For this review, take the finished solid that the model builds, in its own axes (mm). A direction names the side the tool comes from. Round coordinates to 2 decimals unless told otherwise and drop trailing zeros. Loops run counter-clockwise (first coordinate to the right, second up) from the corner with the lowest first, then second, coordinate; pieces in that order, holes last. Notation, with made-up numbers: M 56.25,82.5 L 109.25,82.5 A10 ccw 109.25,89.5 Z; hole C -11,32 d9. An arc over 180 degrees is marked long. Write item = value, one per line. Start each with the question number.
```python
from build123d import *
from build123d import SkipClean  # not in build123d's __all__

# Parameters (mm, degrees)
F0_R      = 19.431
F1_DEPTH  = 2.032
F3_DEPTH  = 5.334
F5_DEPTH  = 14.732
F6_R      = 4.2469525028
F6_R_2    = 2.4689525028
F7_DEPTH  = 14.732
F9_DEPTH  = 2.032
F11_DEPTH = 14.732


# Not quite as in the source:
# - after a boolean that leaves OpenCascade's solid faulty, fix() repairs it


with BuildPart() as f1:
    # F0 (on Top) → F1 (new body)
    with BuildSketch(Plane.XY):
        Circle(F0_R)
    extrude(amount=F1_DEPTH)

    # F2 (on face) → F3 (join)
    with BuildSketch(Plane.XY.offset(2.032)):
        with BuildLine():
            Line((3.937, 3.937), (3.937, 19.0279739331))
            ThreePointArc((3.937, 19.0279739331), (0, 19.431), (-3.937, 19.0279739331))
            Line((-3.937, 19.0279739331), (-3.937, 3.937))
            Line((-3.937, 3.937), (-19.0279739331, 3.937))
            ThreePointArc((-19.0279739331, 3.937), (-19.431, 0), (-19.0279739331, -3.937))
            Line((-19.0279739331, -3.937), (-3.937, -3.937))
            Line((-3.937, -3.937), (-3.937, -19.0279739331))
            ThreePointArc((-3.937, -19.0279739331), (0, -19.431), (3.937, -19.0279739331))
            Line((3.937, -19.0279739331), (3.937, -3.937))
            Line((3.937, -3.937), (19.0279739331, -3.937))
            ThreePointArc((19.0279739331, -3.937), (19.431, 0), (19.0279739331, 3.937))
            Line((19.0279739331, 3.937), (3.937, 3.937))
        make_face()
    extrude(amount=F3_DEPTH)

    # F4 (on face) → F5 (join)
    with BuildSketch(Plane.XY.offset(7.366)):
        with BuildLine():
            ThreePointArc((3.937, 19.0279739331), (3.3670017313, 19.1370598667), (2.794, 19.2290749908))
            Line((2.794, 19.2290749908), (2.794, 2.794))
            Line((2.794, 2.794), (19.2290749908, 2.794))
            ThreePointArc((19.2290749908, 2.794), (19.1370598667, 3.3670017313), (19.0279739331, 3.937))
            ThreePointArc((19.0279739331, 3.937), (18.9302833655, 4.3827083751), (18.822154101, 4.826))
            Line((18.822154101, 4.826), (4.826, 4.826))
            Line((4.826, 4.826), (4.826, 18.822154101))
            ThreePointArc((4.826, 18.822154101), (4.3827083751, 18.9302833655), (3.937, 19.0279739331))
        make_face()
        with BuildLine():
            ThreePointArc((-3.937, 19.0279739331), (-4.3827083751, 18.9302833655), (-4.826, 18.822154101))
            Line((-4.826, 18.822154101), (-4.826, 4.826))
            Line((-4.826, 4.826), (-18.822154101, 4.826))
            ThreePointArc((-18.822154101, 4.826), (-18.9302833655, 4.3827083751), (-19.0279739331, 3.937))
            ThreePointArc((-19.0279739331, 3.937), (-19.1370598667, 3.3670017313), (-19.2290749908, 2.794))
            Line((-19.2290749908, 2.794), (-2.794, 2.794))
            Line((-2.794, 2.794), (-2.794, 19.2290749908))
            ThreePointArc((-2.794, 19.2290749908), (-3.3670017313, 19.1370598667), (-3.937, 19.0279739331))
        make_face()
        with BuildLine():
            ThreePointArc((-19.0279739331, -3.937), (-18.9302833655, -4.3827083751), (-18.822154101, -4.826))
            Line((-18.822154101, -4.826), (-4.826, -4.826))
            Line((-4.826, -4.826), (-4.826, -18.822154101))
            ThreePointArc((-4.826, -18.822154101), (-4.3827083751, -18.9302833655), (-3.937, -19.0279739331))
            ThreePointArc((-3.937, -19.0279739331), (-3.3670017313, -19.1370598667), (-2.794, -19.2290749908))
            Line((-2.794, -19.2290749908), (-2.794, -2.794))
            Line((-2.794, -2.794), (-19.2290749908, -2.794))
            ThreePointArc((-19.2290749908, -2.794), (-19.1370598667, -3.3670017313), (-19.0279739331, -3.937))
        make_face()
        with BuildLine():
            ThreePointArc((3.937, -19.0279739331), (4.3827083751, -18.9302833655), (4.826, -18.822154101))
            Line((4.826, -18.822154101), (4.826, -4.826))
            Line((4.826, -4.826), (18.822154101, -4.826))
            ThreePointArc((18.822154101, -4.826), (18.9302833655, -4.3827083751), (19.0279739331, -3.937))
            ThreePointArc((19.0279739331, -3.937), (19.1370598667, -3.3670017313), (19.2290749908, -2.794))
            Line((19.2290749908, -2.794), (2.794, -2.794))
            Line((2.794, -2.794), (2.794, -19.2290749908))
            ThreePointArc((2.794, -19.2290749908), (3.3670017313, -19.1370598667), (3.937, -19.0279739331))
        make_face()
    extrude(amount=F5_DEPTH)

    # F6 (on face) → F7 (join, through all)
    with BuildSketch(Plane.XY.offset(7.366)):
        Circle(F6_R)
        Circle(F6_R_2, mode=Mode.SUBTRACT)
    extrude(amount=F7_DEPTH)

    # F8 (on face) → F9 (join)
    with BuildSketch(Plane(origin=(0, 0, 7.366), x_dir=(1, 0, 0), z_dir=(0, 0, -1))):
        with BuildLine():
            Line((-3.937, 3.937), (-3.937, 19.0279739331))
            ThreePointArc((-3.937, 19.0279739331), (-13.7397918652, 13.7397918652), (-19.0279739331, 3.937))
            Line((-19.0279739331, 3.937), (-3.937, 3.937))
        make_face()
        with BuildLine():
            ThreePointArc((-19.0279739331, -3.937), (-13.7397918652, -13.7397918652), (-3.937, -19.0279739331))
            Line((-3.937, -19.0279739331), (-3.937, -3.937))
            Line((-3.937, -3.937), (-19.0279739331, -3.937))
        make_face()
        with BuildLine():
            ThreePointArc((3.937, -19.0279739331), (13.7397918652, -13.7397918652), (19.0279739331, -3.937))
            Line((19.0279739331, -3.937), (3.937, -3.937))
            Line((3.937, -3.937), (3.937, -19.0279739331))
        make_face()
        with BuildLine():
            ThreePointArc((19.0279739331, 3.937), (13.7397918652, 13.7397918652), (3.937, 19.0279739331))
            Line((3.937, 19.0279739331), (3.937, 3.937))
            Line((3.937, 3.937), (19.0279739331, 3.937))
        make_face()
    with SkipClean():  # cleaning this boolean's faces spoils the solid; the shape is the same uncleaned
        extrude(amount=F9_DEPTH)

    # F10 (on face) → F11 (join, through all)
    with BuildSketch(Plane.XY.offset(22.098)):
        with BuildLine():
            Line((16.1810749908, -2.794), (17.7050749908, -2.794))
            ThreePointArc((17.7050749908, -2.794), (16.9430749908, -2.032), (16.1810749908, -2.794))
        make_face()
        with BuildLine():
            Line((12.8790749908, -2.794), (14.4030749908, -2.794))
            ThreePointArc((14.4030749908, -2.794), (13.6410749908, -2.032), (12.8790749908, -2.794))
        make_face()
        with BuildLine():
            Line((9.5770749908, -2.794), (11.1010749908, -2.794))
            ThreePointArc((11.1010749908, -2.794), (10.3390749908, -2.032), (9.5770749908, -2.794))
        make_face()
        with BuildLine():
            Line((6.2750749908, -2.794), (7.7990749908, -2.794))
            ThreePointArc((7.7990749908, -2.794), (7.0370749908, -2.032), (6.2750749908, -2.794))
        make_face()
        with BuildLine():
            ThreePointArc((16.1810749908, 2.794), (16.9430749908, 2.032), (17.7050749908, 2.794))
            Line((17.7050749908, 2.794), (16.1810749908, 2.794))
        make_face()
        with BuildLine():
            ThreePointArc((6.2750749908, 2.794), (7.0370749908, 2.032), (7.7990749908, 2.794))
            Line((7.7990749908, 2.794), (6.2750749908, 2.794))
        make_face()
        with BuildLine():
            ThreePointArc((12.8790749908, 2.794), (13.6410749908, 2.032), (14.4030749908, 2.794))
            Line((14.4030749908, 2.794), (12.8790749908, 2.794))
        make_face()
        with BuildLine():
            ThreePointArc((9.5770749908, 2.794), (10.3390749908, 2.032), (11.1010749908, 2.794))
            Line((11.1010749908, 2.794), (9.5770749908, 2.794))
        make_face()
        with BuildLine():
            Line((2.794, 9.5770749908), (2.794, 11.1010749908))
            ThreePointArc((2.794, 11.1010749908), (2.032, 10.3390749908), (2.794, 9.5770749908))
        make_face()
        with BuildLine():
            ThreePointArc((-2.794, 9.5770749908), (-2.032, 10.3390749908), (-2.794, 11.1010749908))
            Line((-2.794, 11.1010749908), (-2.794, 9.5770749908))
        make_face()
        with BuildLine():
            Line((2.794, 6.2750749908), (2.794, 7.7990749908))
            ThreePointArc((2.794, 7.7990749908), (2.032, 7.0370749908), (2.794, 6.2750749908))
        make_face()
        with BuildLine():
            Line((2.794, 16.1810749908), (2.794, 17.7050749908))
            ThreePointArc((2.794, 17.7050749908), (2.032, 16.9430749908), (2.794, 16.1810749908))
        make_face()
        with BuildLine():
            ThreePointArc((-2.794, 16.1810749908), (-2.032, 16.9430749908), (-2.794, 17.7050749908))
            Line((-2.794, 17.7050749908), (-2.794, 16.1810749908))
        make_face()
        with BuildLine():
            ThreePointArc((-2.794, 6.2750749908), (-2.032, 7.0370749908), (-2.794, 7.7990749908))
            Line((-2.794, 7.7990749908), (-2.794, 6.2750749908))
        make_face()
        with BuildLine():
            Line((2.794, 12.8790749908), (2.794, 14.4030749908))
            ThreePointArc((2.794, 14.4030749908), (2.032, 13.6410749908), (2.794, 12.8790749908))
        make_face()
        with BuildLine():
            ThreePointArc((-2.794, 12.8790749908), (-2.032, 13.6410749908), (-2.794, 14.4030749908))
            Line((-2.794, 14.4030749908), (-2.794, 12.8790749908))
        make_face()
        with BuildLine():
            Line((-9.5770749908, 2.794), (-11.1010749908, 2.794))
            ThreePointArc((-11.1010749908, 2.794), (-10.3390749908, 2.032), (-9.5770749908, 2.794))
        make_face()
        with BuildLine():
            ThreePointArc((-9.5770749908, -2.794), (-10.3390749908, -2.032), (-11.1010749908, -2.794))
            Line((-11.1010749908, -2.794), (-9.5770749908, -2.794))
        make_face()
        with BuildLine():
            Line((-6.2750749908, 2.794), (-7.7990749908, 2.794))
            ThreePointArc((-7.7990749908, 2.794), (-7.0370749908, 2.032), (-6.2750749908, 2.794))
        make_face()
        with BuildLine():
            Line((-16.1810749908, 2.794), (-17.7050749908, 2.794))
            ThreePointArc((-17.7050749908, 2.794), (-16.9430749908, 2.032), (-16.1810749908, 2.794))
        make_face()
        with BuildLine():
            ThreePointArc((-16.1810749908, -2.794), (-16.9430749908, -2.032), (-17.7050749908, -2.794))
            Line((-17.7050749908, -2.794), (-16.1810749908, -2.794))
        make_face()
        with BuildLine():
            ThreePointArc((-6.2750749908, -2.794), (-7.0370749908, -2.032), (-7.7990749908, -2.794))
            Line((-7.7990749908, -2.794), (-6.2750749908, -2.794))
        make_face()
        with BuildLine():
            Line((-12.8790749908, 2.794), (-14.4030749908, 2.794))
            ThreePointArc((-14.4030749908, 2.794), (-13.6410749908, 2.032), (-12.8790749908, 2.794))
        make_face()
        with BuildLine():
            ThreePointArc((-12.8790749908, -2.794), (-13.6410749908, -2.032), (-14.4030749908, -2.794))
            Line((-14.4030749908, -2.794), (-12.8790749908, -2.794))
        make_face()
        with BuildLine():
            Line((-2.794, -9.5770749908), (-2.794, -11.1010749908))
            ThreePointArc((-2.794, -11.1010749908), (-2.032, -10.3390749908), (-2.794, -9.5770749908))
        make_face()
        with BuildLine():
            ThreePointArc((2.794, -9.5770749908), (2.032, -10.3390749908), (2.794, -11.1010749908))
            Line((2.794, -11.1010749908), (2.794, -9.5770749908))
        make_face()
        with BuildLine():
            Line((-2.794, -6.2750749908), (-2.794, -7.7990749908))
            ThreePointArc((-2.794, -7.7990749908), (-2.032, -7.0370749908), (-2.794, -6.2750749908))
        make_face()
        with BuildLine():
            Line((-2.794, -16.1810749908), (-2.794, -17.7050749908))
            ThreePointArc((-2.794, -17.7050749908), (-2.032, -16.9430749908), (-2.794, -16.1810749908))
        make_face()
        with BuildLine():
            ThreePointArc((2.794, -16.1810749908), (2.032, -16.9430749908), (2.794, -17.7050749908))
            Line((2.794, -17.7050749908), (2.794, -16.1810749908))
        make_face()
        with BuildLine():
            ThreePointArc((2.794, -6.2750749908), (2.032, -7.0370749908), (2.794, -7.7990749908))
            Line((2.794, -7.7990749908), (2.794, -6.2750749908))
        make_face()
        with BuildLine():
            Line((-2.794, -12.8790749908), (-2.794, -14.4030749908))
            ThreePointArc((-2.794, -14.4030749908), (-2.032, -13.6410749908), (-2.794, -12.8790749908))
        make_face()
        with BuildLine():
            ThreePointArc((2.794, -12.8790749908), (2.032, -13.6410749908), (2.794, -14.4030749908))
            Line((2.794, -14.4030749908), (2.794, -12.8790749908))
        make_face()
    extrude(amount=-F11_DEPTH)

    add(f1.part.fix(), mode=Mode.REPLACE)


solid = f1.part
```
(1) Add section C-C on x = 12. Write out the cut boundary in (y, z).
(2) Tool access review of faces 1 (the flat face through (18, 2.794, 15)), 2 (the flat face through (11, 0, 7.366)), 3 (the flat face through (-10, 10, 7.366)): name each direction out of +Z, -Z, +X, -X, +Y, -Y from which nothing blocks a thin tool from reaching the whole face with its end or side.
(3) For pin 1 Ø12 at (x, y) = (11.5, -12.5) entering from -Z; pin 2 Ø0.9 at (y, z) = (8.5, 17.5) entering from -X; pin 3 Ø0.9 at (y, z) = (-12.5, 18) entering from +X; pin 4 Ø6 at (y, z) = (-6.5, 4.5) entering from -X, all flat-tipped, find the tip position at first contact; note any pin that passes through.
(4) Wall thickness on L1, parallel to Z at x = -7.5, y = 10; L2, parallel to Y at x = -17, z = 21.25; L3, parallel to X at y = 9, z = 10.25: over which ranges is each line inside the solid? List them lowest first.
(5) Add section A-A on x = 0. Write out the cut boundary in (y, z), and give its area (3 significant figures).
(6) Draft analysis for pull direction X (two halves, no side actions). For faces 4 (the cylindrical face through (10.356, -2.032, 14.835)), 5 (the flat face through (10, -10, 5.334)), 6 (the cylindrical face through (16.926, 2.032, 14.835)), 7 (the flat face through (3.937, -12, 4)), state which applies: +X half, -X half, draft (parallel to the pull), parting line (faces both ways), or undercut.
(7) Add section D-D on y = -9. Write out the cut boundary in (x, z).
Answer sheet:
q1.outline = M -15.28,0 L 15.28,0 L 15.28,2.03 L 3.94,2.03 L 3.94,5.33 L 15.28,5.33 L 15.28,7.37 L 4.83,7.37 L 4.83,22.1 L 2.79,22.1 L 2.79,7.37 L -2.79,7.37 L -2.79,22.1 L -4.83,22.1 L -4.83,7.37 L -15.28,7.37 L -15.28,5.33 L -3.94,5.33 L -3.94,2.03 L -15.28,2.03 Z
q2.face_1 = +Z, +X
q2.face_2 = +Z
q2.face_3 = +Z, -X, +Y
q3.pin_1 = 0
q3.pin_2 = -4.83
q3.pin_3 = 4.83
q3.pin_4 = -19.11
q4.L1 = 0 to 2.03, 5.33 to 7.37
q4.L2 = -4.83 to -2.03, 2.03 to 4.83
q4.L3 = -4.83 to -2.79, 2.79 to 4.83
q5.outline = M -19.43,0 L 19.43,0 L 19.43,7.37 L 4.25,7.37 L 4.25,22.1 L 2.47,22.1 L 2.47,7.37 L -2.47,7.37 L -2.47,22.1 L -4.25,22.1 L -4.25,7.37 L -19.43,7.37 Z
q5.area = 339 mm²
q6.face_4 = undercut
q6.face_5 = draft
q6.face_6 = undercut
q6.face_7 = +X half
q7.outline = M -17.22,0 L 17.22,0 L 17.22,2.03 L 3.94,2.03 L 3.94,5.33 L 17.22,5.33 L 17.22,7.37 L 4.83,7.37 L 4.83,22.1 L 2.79,22.1 L 2.79,7.37 L -2.79,7.37 L -2.79,22.1 L -4.83,22.1 L -4.83,7.37 L -17.22,7.37 L -17.22,5.33 L -3.94,5.33 L -3.94,2.03 L -17.22,2.03 Z
